```python
from build123d import *

# Parameters (mm, degrees)
SKETCH1_R           = 1.5
BOSS_EXTRUDE1_DEPTH = 2.4


with BuildPart() as part:
    # Sketch1 → Boss-Extrude1 (new body)
    with BuildSketch(Plane.XY):
        with BuildLine():
            Line((2.547107201, 13.777973489), (2.60207137, 13.767698905))
            ThreePointArc((2.60207137, 13.767698905), (2.893171321, 13.597662774), (3.010168721, 13.281493396))
            Line((3.010168721, 13.281493396), (3.021754222, 12.184659018))
            ThreePointArc((3.021754222, 12.184659018), (3.435499758, 12.074529199), (3.845249182, 11.950354501))
            Line((3.845249182, 11.950354501), (4.432508267, 12.876802904))
            ThreePointArc((4.432508267, 12.876802904), (4.698423191, 13.084024332), (5.035433845, 13.075347588))
            Line((5.035433845, 13.075347588), (5.087574195, 13.055148308))
            ThreePointArc((5.087574195, 13.055148308), (5.342473559, 12.83451789), (5.399382885, 12.502233681))
            Line((5.399382885, 12.502233681), (5.209228333, 11.421946163))
            ThreePointArc((5.209228333, 11.421946163), (5.595692764, 11.23766597), (5.975648384, 11.040314323))
            Line((5.975648384, 11.040314323), (6.723142715, 11.843079608))
            ThreePointArc((6.723142715, 11.843079608), (7.02260677, 11.997910958), (7.35228483, 11.927456407))
            Line((7.35228483, 11.927456407), (7.399825783, 11.898020294))
            ThreePointArc((7.399825783, 11.898020294), (7.609844268, 11.634308893), (7.604727542, 11.297225393))
            Line((7.604727542, 11.297225393), (7.219308422, 10.27027263))
            ThreePointArc((7.219308422, 10.27027263), (7.565331165, 10.018117505), (7.902554048, 9.754309483))
            Line((7.902554048, 9.754309483), (8.784828602, 10.406054439))
            ThreePointArc((8.784828602, 10.406054439), (9.107643898, 10.503223117), (9.418762572, 10.373390003))
            Line((9.418762572, 10.373390003), (9.460085179, 10.335719469))
            ThreePointArc((9.460085179, 10.335719469), (9.618070857, 10.03790746), (9.551102323, 9.707503643))
            Line((9.551102323, 9.707503643), (8.98354362, 8.76885728))
            ThreePointArc((8.98354362, 8.76885728), (9.277341286, 8.457414063), (9.560347713, 8.136133332))
            Line((9.560347713, 8.136133332), (10.547357686, 8.614663568))
            ThreePointArc((10.547357686, 8.614663568), (10.882531136, 8.650860609), (11.164495652, 8.466070244))
            Line((11.164495652, 8.466070244), (11.198192721, 8.421448114))
            ThreePointArc((11.198192721, 8.421448114), (11.298765579, 8.099677128), (11.172225769, 7.7872045))
            Line((11.172225769, 7.7872045), (10.441855016, 6.968829012))
            ThreePointArc((10.441855016, 6.968829012), (10.673422677, 6.608703529), (10.892575202, 6.240890918))
            Line((10.892575202, 6.240890918), (11.950709155, 6.529910661))
            ThreePointArc((11.950709155, 6.529910661), (12.286826829, 6.503903419), (12.530035223, 6.270448618))
            Line((12.530035223, 6.270448618), (12.55495924, 6.220394444))
            ThreePointArc((12.55495924, 6.220394444), (12.594694391, 5.885622006), (12.412892467, 5.601721447))
            Line((12.412892467, 5.601721447), (11.544581562, 4.931485631))
            ThreePointArc((11.544581562, 4.931485631), (11.70603346, 4.534941522), (11.853869106, 4.133122449))
            Line((11.853869106, 4.133122449), (12.947093557, 4.222789479))
            ThreePointArc((12.947093557, 4.222789479), (13.27270937, 4.135463598), (13.468879472, 3.861294384))
            Line((13.468879472, 3.861294384), (13.48418168, 3.807512701))
            ThreePointArc((13.48418168, 3.807512701), (13.461725991, 3.471139085), (13.230852999, 3.225478489))
            Line((13.230852999, 3.225478489), (12.254171229, 2.726206422))
            ThreePointArc((12.254171229, 2.726206422), (12.340009313, 2.306747521), (12.411493716, 1.884605453))
            Line((12.411493716, 1.884605453), (13.502580216, 1.771866265))
            ThreePointArc((13.502580216, 1.771866265), (13.806605713, 1.626195525), (13.949057185, 1.320648401))
            Line((13.949057185, 1.320648401), (13.954216486, 1.26497068))
            ThreePointArc((13.954216486, 1.26497068), (13.870334657, 0.938450687), (13.598252701, 0.73939573))
            Line((13.598252701, 0.73939573), (12.546459793, 0.428089522))
            ThreePointArc((12.546459793, 0.428089522), (3.253260702, -12.124900362), (-11.075595423, -5.91))
            Line((-11.075595423, -5.91), (-31.235799276, -5.175527107))
            ThreePointArc((-31.235799276, -5.175527107), (-34.653079748, -3.649418925), (-36.053760949, -0.178842001))
            Line((-36.053760949, -0.178842001), (-36.053760949, 0.178842001))
            ThreePointArc((-36.053760949, 0.178842001), (-34.653079748, 3.649418925), (-31.235799276, 5.175527107))
            Line((-31.235799276, 5.175527107), (-11.075595423, 5.91))
            ThreePointArc((-11.075595423, 5.91), (-6.768701925, 10.572681222), (-0.731377895, 12.532437925))
            Line((-0.731377895, 12.532437925), (-0.518446871, 13.608467783))
            ThreePointArc((-0.518446871, 13.608467783), (-0.345345603, 13.89775556), (-0.027958125, 14.011407027))
            Line((-0.027958125, 14.011407027), (0.027958125, 14.011407027))
            ThreePointArc((0.027958125, 14.011407027), (0.345345603, 13.89775556), (0.518446871, 13.608467783))
            Line((0.518446871, 13.608467783), (0.731377895, 12.532437925))
            ThreePointArc((0.731377895, 12.532437925), (1.158314928, 12.500208818), (1.58390463, 12.453439689))
            Line((1.58390463, 12.453439689), (1.990930066, 13.472022121))
            ThreePointArc((1.990930066, 13.472022121), (2.214240445, 13.72457695), (2.547107201, 13.777973489))
        make_face()
        with Locations((6.276880475, 0)):
            Circle(SKETCH1_R, mode=Mode.SUBTRACT)
        with Locations((-6.276880475, 0)):
            Circle(SKETCH1_R, mode=Mode.SUBTRACT)
        Circle(SKETCH1_R, mode=Mode.SUBTRACT)
        with Locations((-31.235799276, 0)):
            Circle(SKETCH1_R, mode=Mode.SUBTRACT)
    extrude(amount=BOSS_EXTRUDE1_DEPTH)


solid = part.part
```
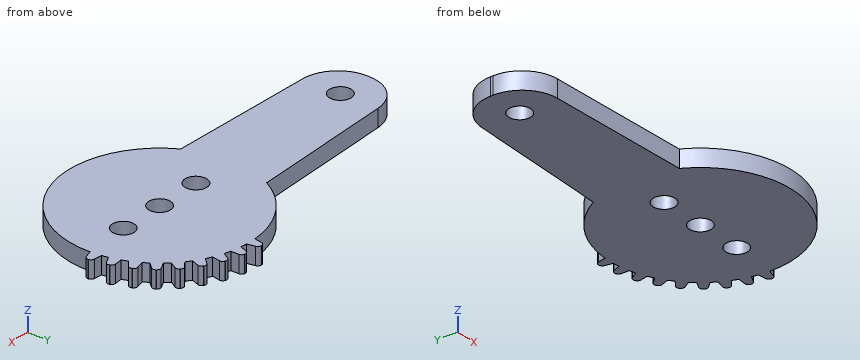
The listing builds one solid part. Answer for the finished solid, in the listing's coordinates (mm). Coordinates: 2 decimals unless noted, no trailing zeros. Loops run counter-clockwise (first coordinate to the right, second up) from the corner with the lowest first, then second, coordinate; pieces in that order, holes last. Notation, with made-up numbers: M -36.75,52.5 L 1.25,52.5 A14 cw 1.25,62.5 Z; hole C 29.5,-35 d9. An arc over 180 degrees is marked long. Answer as a JSON object with one key per item and string values. Group by question number.
Item 1: Section C-C (x = -20) is taken. Write down the section's boundary in (y, z), and give its area (3 significant figures).
Item 2: This flat-tipped pin is pushed along its axis until it touches: P1, Ø1, axis at x = -10.5, z = 1.5, coming from the -Y side. Where does it stop, or does it pass through?
Item 3: Section B-B (x = -25.5) is taken. Write down the section's boundary in (y, z), and give its area (3 significant figures).
Item 4: Consider L1, parallel to X at y = 8.5, z = 0.3; L2, parallel to Y at x = -9.5, z = 0.4; L3, parallel to X at y = 10, z = 2.15. Determine where each line is inside the solid, lowest interval first.
Item 5: Section A-A (z = 0.55) is taken. Give the number of separate pieces and of enclosed holes in the cut face, and give its area (3 significant figures).
Solved:
{
 "1": {"outline": "M -5.58,0 L 5.58,0 L 5.58,2.4 L -5.58,2.4 Z", "area": "26.8 mm2"},
 "2": {"P1": "stops at y = -7.59"},
 "3": {"outline": "M -5.38,0 L 5.38,0 L 5.38,2.4 L -5.38,2.4 Z", "area": "25.8 mm2"},
 "4": {"L1": "x = -9.24 to 9.24, 10.31 to 11.14", "L2": "y = -8.21 to 8.21", "L3": "x = -7.59 to 7.59, 8.24 to 9.62"},
 "5": {"separate pieces": "1", "enclosed holes": "4", "area": "732 mm2"}
}
